Design review of the part built by this model. Coordinates are the model's own, in mm. Face numbers are marked on the shaded views. Give positions to 0.01 mm unless a question says otherwise; leave off trailing zeros. Order: outer loops, then holes, each group sorted by start corner. A loop starts at its lowest first (then second) coordinate and runs counter-clockwise, first axis right, second up. Notation, with made-up numbers: (39, 87.25) -> (63, 87.25) arc R16 cw to (63, 103.25) -> close; hole circle Ø6 at (5, 27). An arc over 180 degrees is marked (long way). Answer in a Markdown table with one row per item. Add a question column.
```python
from build123d import *

# Parameters (mm, degrees)
F0_R     = 2
F1_DEPTH = 3
F2_R     = 5
F2_R_2   = 2
F3_DEPTH = 1
F5_R     = 0.2


# Not quite as in the source:
# - a fillet or chamfer that OpenCascade refuses, or shapes differently, is made with other operations: its cross-section is extruded or revolved along the edge and cut away or added


with BuildPart() as f1:
    # F0 (on Top) → F1 (new body)
    with BuildSketch(Plane.XY):
        Polygon((1.5066089403, -4.3661725612), (4.5345208255, -0.8783246648), (3.0279118852, 3.4878478965), (-1.5066089403, 4.3661725612), (-4.5345208255, 0.8783246648), (-3.0279118852, -3.4878478965), align=None)
        Circle(F0_R, mode=Mode.SUBTRACT)
    extrude(amount=F1_DEPTH)

    # F2 (on face) → F3 (join)
    with BuildSketch(Plane.XY.offset(3)):
        Circle(F2_R)
        Circle(F2_R_2, mode=Mode.SUBTRACT)
    extrude(amount=F3_DEPTH)

    # F4: chamfer of 0.4 on 1 edges, made by hand


with BuildPart() as f4_tool2:
    # F4_s3 → F4_t4 (revolve)
    with BuildSketch(Plane.XZ):
        Polygon((4.6, 3), (5, 3.4), (5, 3), align=None)
    revolve(axis=Axis((0, 0, 3), (0, 0, 1)))

    split(bisect_by=Plane(origin=(3.7812163553, 1.3047616158, 0), x_dir=(0, 0, 1), z_dir=(0.9453040888, 0.326190404, 0)), keep=Keep.TOP)


with BuildPart() as f1_1:
    add(f1.part)

    # F4_t1: cut F4_tool2
    add(f4_tool2.part, mode=Mode.SUBTRACT)


with BuildPart() as f4_tool7:
    # F4_s8 → F4_t9 (revolve)
    with BuildSketch(Plane.XZ):
        Polygon((4.6, 3), (5, 3.4), (5, 3), align=None)
    revolve(axis=Axis((0, 0, 3), (0, 0, 1)))

    split(bisect_by=Plane(origin=(0.7606514725, 3.9270102288, 0), x_dir=(0, 0, 1), z_dir=(0.1901628681, 0.9817525572, 0)), keep=Keep.TOP)


with BuildPart() as f1_2:
    add(f1_1.part)

    # F4_t6: cut F4_tool7
    add(f4_tool7.part, mode=Mode.SUBTRACT)


with BuildPart() as f4_tool12:
    # F4_s13 → F4_t14 (revolve)
    with BuildSketch(Plane.XZ):
        Polygon((4.6, 3), (5, 3.4), (5, 3), align=None)
    revolve(axis=Axis((0, 0, 3), (0, 0, 1)))

    split(bisect_by=Plane(origin=(3.0205648829, -2.622248613, 0), x_dir=(0, 0, 1), z_dir=(0.7551412207, -0.6555621532, 0)), keep=Keep.TOP)


with BuildPart() as f1_3:
    add(f1_2.part)

    # F4_t11: cut F4_tool12
    add(f4_tool12.part, mode=Mode.SUBTRACT)


with BuildPart() as f4_tool17:
    # F4_s18 → F4_t19 (revolve)
    with BuildSketch(Plane.XZ):
        Polygon((4.6, 3), (5, 3.4), (5, 3), align=None)
    revolve(axis=Axis((0, 0, 3), (0, 0, 1)))

    split(bisect_by=Plane(origin=(-3.0205648829, 2.622248613, 0), x_dir=(0, 0, 1), z_dir=(-0.7551412207, 0.6555621532, 0)), keep=Keep.TOP)


with BuildPart() as f1_4:
    add(f1_3.part)

    # F4_t16: cut F4_tool17
    add(f4_tool17.part, mode=Mode.SUBTRACT)


with BuildPart() as f4_tool22:
    # F4_s23 → F4_t24 (revolve)
    with BuildSketch(Plane.XZ):
        Polygon((4.6, 3), (5, 3.4), (5, 3), align=None)
    revolve(axis=Axis((0, 0, 3), (0, 0, 1)))

    split(bisect_by=Plane(origin=(-0.7606514725, -3.9270102288, 0), x_dir=(0, 0, 1), z_dir=(-0.1901628681, -0.9817525572, 0)), keep=Keep.TOP)


with BuildPart() as f1_5:
    add(f1_4.part)

    # F4_t21: cut F4_tool22
    add(f4_tool22.part, mode=Mode.SUBTRACT)


with BuildPart() as f4_tool27:
    # F4_s28 → F4_t29 (revolve)
    with BuildSketch(Plane.XZ):
        Polygon((4.6, 3), (5, 3.4), (5, 3), align=None)
    revolve(axis=Axis((0, 0, 3), (0, 0, 1)))

    split(bisect_by=Plane(origin=(-3.7812163553, -1.3047616158, 0), x_dir=(0, 0, 1), z_dir=(-0.9453040888, -0.326190404, 0)), keep=Keep.TOP)


with BuildPart() as f1_6:
    add(f1_5.part)

    # F4_t26: cut F4_tool27
    add(f4_tool27.part, mode=Mode.SUBTRACT)

    # F5
    f5_edges = [f1_6.edges().sort_by_distance(p)[0] for p in [
        (-5, 0, 4),
    ]]
    fillet(f5_edges, radius=F5_R)


solid = f1_6.part
```
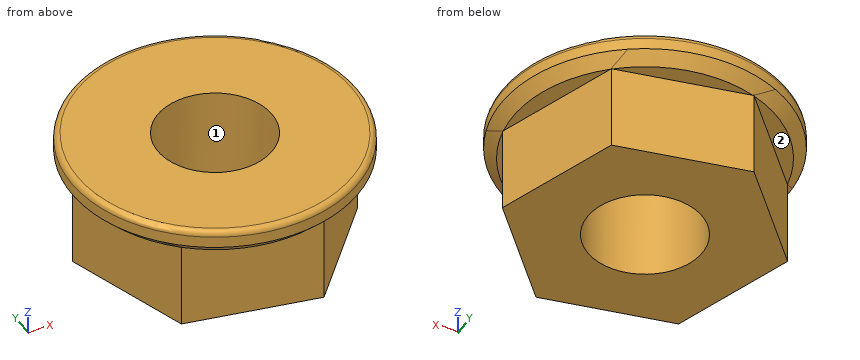
1) Add section C-C, the plane x = 0. Write out the cut boundary in (y, z), and give its area (3 significant figures).
2) Add section D-D, the plane z = 3.65. Write out the cut boundary in (x, y), and give its area (3 significant figures).
3) Clearance check with flat-ended pins moving along their axes: P1, Ø3.5, axis at x = 4, y = -2, coming from the -Z side; P2, Ø1, axis at y = -2.5, z = 3, coming from the -X side; P3, Ø1, axis at y = -2.5, z = 0.5, coming from the -X side; P4, Ø0.5, axis at x = 4, y = 2.5, coming from the -Z side. State where each tip first meets the part, or that it passes through.
4) For L1, parallel to X at y = -0.25, z = 2; L2, parallel to Y at x = -1.25, z = 2.15; L3, parallel to Y at x = 0, z = 1.25, list the stretches that pass through material, from the lowest coordinate up.
5) Add section A-A, the plane z = 0.5. Write out the cut boundary in (x, y).
6) Mouldability with a two-part tool opening along X and no side actions: class the marked faces 1 and 2 as +X half, -X half, draft (parallel to the pull), parting line (faces both ways), or undercut.
7) Add section B-B, the plane y = 0. Write out the cut boundary in (x, z).
Verdict:
| question | item | result |
|---|---|---|
| 1 | outline | (-5, 3.4) -> (-4.6, 3) -> (-4.07, 3) -> (-4.07, 0) -> (-2, 0) -> (-2, 4) -> (-4.8, 4) arc R0.2 ccw to (-5, 3.8) -> close; (2, 0) -> (4.07, 0) -> (4.07, 3) -> (4.6, 3) -> (5, 3.4) -> (5, 3.8) arc R0.2 ccw to (4.8, 4) -> (2, 4) -> close |
| 1 | area | 18.3 mm2 |
| 2 | outline | circle Ø10 at (0, 0); hole circle Ø4 at (0, 0) |
| 2 | area | 66.0 mm2 |
| 3 | P1 | stops at z = 0 |
| 3 | P2 | stops at x = -4.49 |
| 3 | P3 | stops at x = -3.54 |
| 3 | P4 | stops at z = 3 |
| 4 | L1 | x = -4.15 to -1.98, 1.98 to 4.32 |
| 4 | L2 | y = -3.83 to -1.56, 1.56 to 4.32 |
| 4 | L3 | y = -4.07 to -2, 2 to 4.07 |
| 5 | outline | (-4.53, 0.88) -> (-3.03, -3.49) -> (1.51, -4.37) -> (4.53, -0.88) -> (3.03, 3.49) -> (-1.51, 4.37) -> close; hole circle Ø4 at (0, 0) |
| 6 | face 1 | undercut |
| 6 | face 2 | draft |
| 7 | outline | (-5, 3.4) -> (-4.6, 3) -> (-4.23, 3) -> (-4.23, 0) -> (-2, 0) -> (-2, 4) -> (-4.8, 4) arc R0.2 ccw to (-5, 3.8) -> close; (2, 0) -> (4.23, 0) -> (4.23, 3) -> (4.6, 3) -> (5, 3.4) -> (5, 3.8) arc R0.2 ccw to (4.8, 4) -> (2, 4) -> close |
